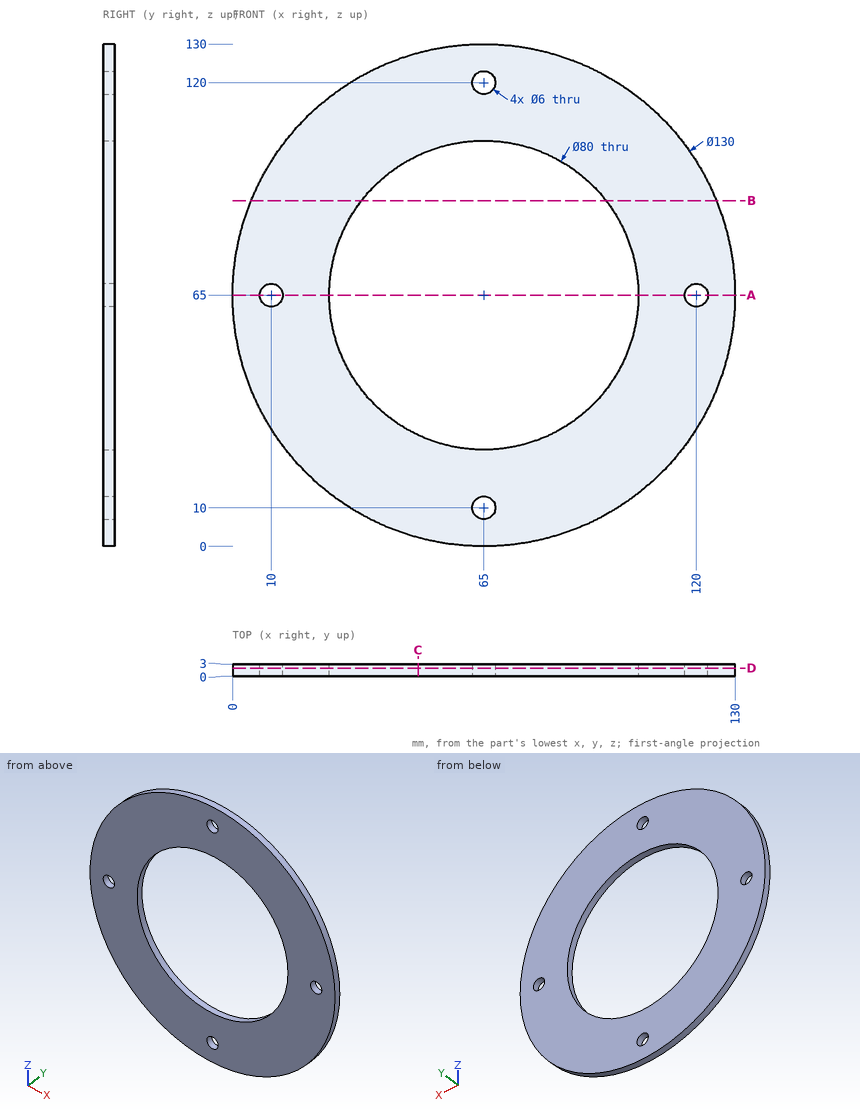
Drawing for the job (mm, zero at the part's lowest x, y, z). Coordinates: 2 decimals unless noted, no trailing zeros. Order: outer loops, then holes, each group sorted by start corner. A loop starts at its lowest first (then second) coordinate and runs counter-clockwise, first axis right, second up. Notation, with made-up numbers: (38, 88.5) - (92, 88.5) arc R24 cw to (92, 115.5) - close; hole circle Ø7 at (-24, -28). An arc over 180 degrees is marked (long way). Use a Markdown table: item, result. Add a question column.
(1) Saw through at A-A (z = 65). Give the cut face in (x, y).
(2) Saw through at B-B (z = 89.5). Give the cut face in (x, y), then the cut area to 3 significant figures.
(3) Saw through at C-C (x = 48). Give the cut face in (y, z).
(4) Flat gauge pin, fed straight in: pin 1 (1 mm diameter, centred on y = 1, z = 39, fed in from -X). Where does the tip first touch, or does it go through?
(5) Saw through at D-D (y = 2.05). Give the cut face in (x, z), then the cut area to 3 significant figures.
(6) Drill centre lines: line 1 along X through (y, z) = (0.9, 65); line 2 along X through (y, z) = (2.05, 81.5). Where is each one in solid material? Low to high. Write a range as [from, to].
Solved:
| question | item | result |
|---|---|---|
| 1 | outline | (0, 0) - (7, 0) - (7, 3) - (0, 3) - close; (13, 0) - (25, 0) - (25, 3) - (13, 3) - close; (105, 0) - (117, 0) - (117, 3) - (105, 3) - close; (123, 0) - (130, 0) - (130, 3) - (123, 3) - close |
| 2 | outline | (4.79, 0) - (33.38, 0) - (33.38, 3) - (4.79, 3) - close; (96.62, 0) - (125.21, 0) - (125.21, 3) - (96.62, 3) - close |
| 2 | area | 172 mm² |
| 3 | outline | (0, 2.26) - (3, 2.26) - (3, 28.79) - (0, 28.79) - close; (0, 101.21) - (3, 101.21) - (3, 127.74) - (0, 127.74) - close |
| 4 | pin 1 | stops at x = 5.21 |
| 5 | outline | circle Ø130 at (65, 65); hole circle Ø6 at (10, 65); hole circle Ø80 at (65, 65); hole circle Ø6 at (65, 10); hole circle Ø6 at (65, 120); hole circle Ø6 at (120, 65) |
| 5 | area | 8,130 mm² |
| 6 | line 1 | x = [0, 7], [13, 25], [105, 117], [123, 130] |
| 6 | line 2 | x = [2.13, 28.56], [101.44, 127.87] |
